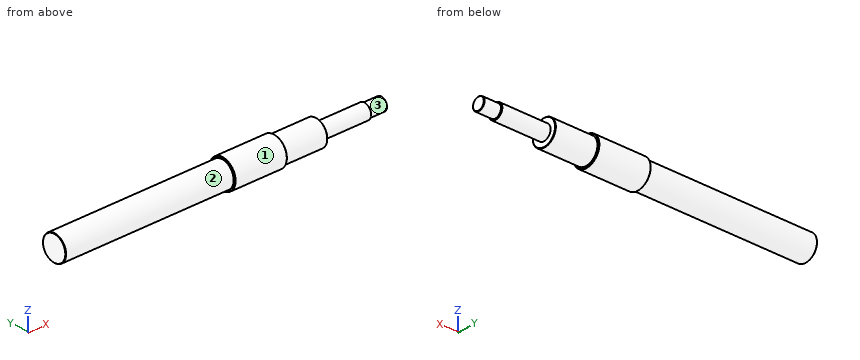
from build123d import *

# Parameters (mm, degrees)
CHAMFER1_SIZE = 0.1


with BuildPart() as part:
    # Sketch1 → Revolve1 (revolve)
    with BuildSketch(Plane.XY, mode=Mode.PRIVATE) as revolve1_sk:
        Polygon((-25.6, 3), (-15.6, 3), (-15.6, 1.75), (-4, 1.75), (-4, 1.5), (0, 1.5), (0, 0), (-78, 0), (-78, 3), (-38, 3), (-38, 3.4), (-25.6, 3.4), align=None)
    revolve(revolve1_sk.sketch.rotate(Axis((0, 0, 0), (1, 0, 0)), 90), axis=Axis((0, 0, 0), (1, 0, 0)))

    # Chamfer1
    chamfer1_edges = [part.edges().sort_by_distance(p)[0] for p in [
        (-4, 0, -1.75),
        (-15.6, 0, -3),
        (-25.6, 0, -3.4),
        (-38, 0, -3.4),
        (-78, 0, -3),
        (0, 0, -1.5),
    ]]
    chamfer(chamfer1_edges, length=CHAMFER1_SIZE)


solid = part.part
Build history of the part. All positions in model axes, mm. Face numbers are marked on the shaded views. A direction names the side the tool comes from. Give positions to 0.01 mm unless a question says otherwise; leave off trailing zeros. Order: outer loops, then holes, each group sorted by start corner. A loop starts at its lowest first (then second) coordinate and runs counter-clockwise, first axis right, second up. Notation, with made-up numbers: M -12,37 L -3,37 A23 ccw -3,67 Z; hole C 38,6 d7. An arc over 180 degrees is marked long. Use one line per item in the form item = value.
1) Saw through at C-C (x = -53). Give the cut face in (y, z), plus the area to 3 significant figures.
Calculated:
outline = C 0,0 d6
area = 28.3 mm2
2) Saw through at D-D (x = -9.5). Give the cut face in (y, z).
Calculated:
outline = C 0,0 d3.5
3) Tool access for the marked faces 1, 2 and 3: list every direction of +Z, -Z, +X, -X, +Y, -Y with a clear straight run to the whole face (end or side of a thin tool).
Calculated:
face_1 = +X, -X
face_2 = -X
face_3 = +X
4) Probe probe 1 along X at (y, z) = (1.5, 1); probe 2 along Y at (x, z) = (-52, -2.5); probe 3 along Y at (x, z) = (-70, 0.25). List the from-to ranges inside material, lowest first.
Calculated:
probe_1 = -78 to -15.6
probe_2 = -1.66 to 1.66
probe_3 = -2.99 to 2.99
5) Drop flat-ended pins along their axis: pin 1 (2.5 mm diameter, centred on y = 0, z = -0.5, fed in from +X); pin 2 (4 mm diameter, centred on x = -13, y = 1, fed in from +Z); pin 3 (1 mm diameter, centred on x = -49, z = -1, fed in from +Y); pin 4 (1.5 mm diameter, centred on x = -16, z = -1, fed in from -Y). Give the stop position or say it passes through.
Calculated:
pin_1 = 0
pin_2 = 1.75
pin_3 = 2.96
pin_4 = -2.99
